Input: part model. Units: mm. Frame: model coordinates. Round coordinates to 2 decimals unless told otherwise and drop trailing zeros. Write each loop counter-clockwise with the first axis right and the second up, starting at its lowest first coordinate (ties: lowest second). Pieces come first, ordered by that corner, then holes. Notation, with made-up numbers: (65, -28.75) -> (109, -28.75) arc R24 cw to (109, 4.25) -> close; hole circle Ø5 at (16, -23.75). An arc over 180 degrees is marked (long way). Write item = value, one per line.
```python
from build123d import *

# Parameters (mm, degrees)
SKETCH1_R           = 1.778
SKETCH1_R_2         = 4.7625
SKETCH1_R_3         = 10.795
BOSS_EXTRUDE1_DEPTH = 1.905


with BuildPart() as part:
    # Sketch1 → Boss-Extrude1 (new body)
    with BuildSketch(Plane(origin=(0, 0, 0), x_dir=(1, 0, 0), z_dir=(0, 1, 0))):
        with BuildLine():
            ThreePointArc((-3.434964073, 4.439030494), (-4.439030494, -3.434964073), (3.434964073, -4.439030494))
            ThreePointArc((3.434964073, -4.439030494), (20.136115591, 6.903606124), (38.111342378, 16.094639222))
            ThreePointArc((38.111342378, 16.094639222), (73.570878275, 13.084704733), (90.4875, -18.2245))
            ThreePointArc((90.4875, -18.2245), (103.1875, -30.9245), (115.8875, -18.2245))
            ThreePointArc((115.8875, -18.2245), (132.804121725, 13.084704733), (168.263657622, 16.094639222))
            ThreePointArc((168.263657622, 16.094639222), (186.238884409, 6.903606124), (202.940035927, -4.439030494))
            ThreePointArc((202.940035927, -4.439030494), (210.814030494, -3.434964073), (209.809964073, 4.439030494))
            ThreePointArc((209.809964073, 4.439030494), (103.1875, 40.874472361), (-3.434964073, 4.439030494))
        make_face()
        with Locations(Location((0, 0, 0), (0, 0, 90))):
            Circle(SKETCH1_R, mode=Mode.SUBTRACT)
        with Locations(Location((206.375, 0, 0), (0, 0, 90))):
            Circle(SKETCH1_R, mode=Mode.SUBTRACT)
        with Locations(Location((103.1875, -18.2245, 0), (0, 0, 90))):
            Circle(SKETCH1_R_2, mode=Mode.SUBTRACT)
        with Locations(Location((103.1875, 19.8755, 0), (0, 0, 90))):
            Circle(SKETCH1_R_3, mode=Mode.SUBTRACT)
    extrude(amount=BOSS_EXTRUDE1_DEPTH)


solid = part.part
```
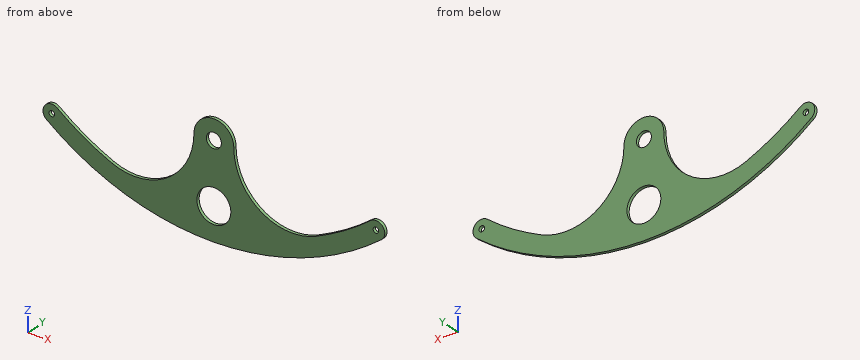
1) Cut plane C-C (z = 25.5). Return the cut outline in (x, y) (3 decimals), and give its area (3 significant figures).
Solutions:
outline = (92.778, 0) -> (113.597, 0) -> (113.597, 1.905) -> (92.778, 1.905) -> close
area = 39.7 mm^2
2) Cut plane B-B (x = 181.5). Return the cut outline in (y, z) (3 decimals).
Solutions:
outline = (0, -22.282) -> (1.905, -22.282) -> (1.905, -9.604) -> (0, -9.604) -> close
3) First-contact query: P1, Ø3, axis at x = 0, z = 0, coming from the -Y side; P2, Ø1, axis at x = 185, y = 0.5, coming from the +Z side. Flat tips, straight axial feed; report the tip coordinate or a pass-through.
Solutions:
P1 = through
P2 = -7.34
4) Line query: L1, parallel to X at y = 1.3, z = -0.5; L2, parallel to X at y = 1.75, z = 0; L3, parallel to X at y = 1.6, z = -7.5. Output: solid intervals per line, ascending. Write a range as from..to.
Solutions:
L1 = -5.59..-1.71, 1.71..10.17, 85.47..120.91, 196.21..204.67, 208.08..211.97
L2 = -5.61..-1.78, 1.78..9.45, 85.75..120.62, 196.92..204.6, 208.15..211.99
L3 = 0.64..21.15, 80.25..126.13, 185.22..205.73
5) Cut plane A-A (y = 0.9). Count the separate pieces of the cut face and the enclosed holes in it, and give its area (3 significant figures).
Solutions:
separate_pieces = 1
enclosed_holes = 4
area = 4,750 mm^2
